Read the model definition and answer for the solid it produces. Units are mm, in the model's axes. Face numbers are marked on the shaded views. A direction names the side the tool comes from. Coordinates: 2 decimals unless noted, no trailing zeros. Loops run counter-clockwise (first coordinate to the right, second up) from the corner with the lowest first, then second, coordinate; pieces in that order, holes last. Notation, with made-up numbers: (19, -37.5) -> (60, -37.5) arc R23 cw to (60, -29.5) -> close; hole circle Ø10 at (33, 67.5). An arc over 180 degrees is marked (long way). One line per question, with ' | ' between items. Start each with the question number.
```python
from build123d import *

# Parameters (mm, degrees)
SKETCH_2_W          = 50
SKETCH_2_H          = 25
EXTRUDE_4_DEPTH     = 5
SKETCH_7_W          = 50
SKETCH_7_H          = 5
EXTRUDE_5_DEPTH     = 40.339506062
FILLET_11_R         = 2
FILLET_12_R         = 2
FILLET_15_R         = 5
FILLET_17_R         = 2
FILLET_18_R         = 2
FILLET_19_R         = 2
SKETCH_8_R          = 8.1
CUT_EXTRUDE_4_DEPTH = 25


with BuildPart() as part:
    # 草图2 → 凸台-拉伸4 (new body)
    with BuildSketch(Plane(origin=(0, 0, 0), x_dir=(1, 0, 0), z_dir=(0, 1, 0))):
        with Locations((25, 12.5)):
            Rectangle(SKETCH_2_W, SKETCH_2_H)
    extrude(amount=EXTRUDE_4_DEPTH)

    # 草图7 → 凸台-拉伸5 (add)
    with BuildSketch(Plane(origin=(0, 5, 0), x_dir=(1, 0, 0), z_dir=(0, 1, 0))):
        with Locations((25, 2.5)):
            Rectangle(SKETCH_7_W, SKETCH_7_H)
    extrude(amount=EXTRUDE_5_DEPTH)

    # 圆角11
    fillet_11_edges = [part.edges().sort_by_distance(p)[0] for p in [
        (25, 45.339506062, 0),
    ]]
    fillet(fillet_11_edges, radius=FILLET_11_R)

    # 圆角12
    fillet_12_edges = [part.edges().sort_by_distance(p)[0] for p in [
        (25, 45.339506062, -5),
    ]]
    fillet(fillet_12_edges, radius=FILLET_12_R)

    # 圆角15
    fillet_15_edges = [part.edges().sort_by_distance(p)[0] for p in [
        (25, 5, -5),
    ]]
    fillet(fillet_15_edges, radius=FILLET_15_R)

    # 圆角17
    fillet_17_edges = [part.edges().sort_by_distance(p)[0] for p in [
        (50, 45.339506062, -2.5),
        (50, 21.669753031, 0),
        (50, 44.753719625, -0.585786438),
        (50, 26.669753031, -5),
        (50, 44.753719625, -4.414213562),
        (50, 5, -17.5),
        (50, 6.464466094, -6.464466094),
        (50, 0, -12.5),
        (50, 2.5, -25),
    ]]
    fillet(fillet_17_edges, radius=FILLET_17_R)

    # 圆角18
    # the kernel refuses this fillet: 2 mm, written as the material it takes off along each edge
    with BuildSketch(Plane(origin=(48, 3, -23), x_dir=(0, 0, -1), z_dir=(0, 1, 0))) as fillet_18_piece_1_section:
        Polygon((0, 0), (FILLET_18_R, 0), (FILLET_18_R, -FILLET_18_R), (0, -FILLET_18_R), align=None)
    fillet_18_piece_1 = extrude(amount=FILLET_18_R, mode=Mode.PRIVATE)
    fillet_18_piece_1 = fillet_18_piece_1 - Plane(origin=(48, 3, -23), x_dir=(-0.7071067811865475, 0, 0.7071067811865475), z_dir=(0, 1, 0)) * Sphere(FILLET_18_R, mode=Mode.PRIVATE)
    add(fillet_18_piece_1, mode=Mode.SUBTRACT)
    with BuildSketch(Plane(origin=(48, 5, -25), x_dir=(0, 0, 1), z_dir=(-1, 0, 0))) as fillet_18_piece_2:
        with BuildLine():
            CenterArc((FILLET_18_R, -FILLET_18_R), FILLET_18_R, 90, 90)
            Line((0, -FILLET_18_R), (0, 0))
            Line((0, 0), (FILLET_18_R, 0))
        make_face()
    extrude(amount=53, mode=Mode.SUBTRACT)

    # 圆角19
    fillet_19_edges = [part.edges().sort_by_distance(p)[0] for p in [
        (0, 21.669753031, 0),
        (0, 44.753719625, -0.585786438),
        (0, 45.339506062, -2.5),
        (0, 26.669753031, -5),
        (0, 44.753719625, -4.414213562),
        (0, 6.464466094, -6.464466094),
        (0, 0, -12.5),
        (0, 5, -16.5),
        (0, 1.5, -25),
        (0, 4.414213562, -24.414213562),
    ]]
    fillet(fillet_19_edges, radius=FILLET_19_R)

    # 草图8 → 切除-拉伸4 (cut)
    with BuildSketch(Plane(origin=(0, 0, -5), x_dir=(-1, 0, 0), z_dir=(0, 0, -1))):
        with Locations(Location((-37.5, 35.339506062, 0), (0, 0, 80.987548501))):
            Circle(SKETCH_8_R)
        with Locations(Location((-12.5, 35.339506062, 0), (0, 0, 80.987548501))):
            Circle(SKETCH_8_R)
    extrude(amount=-CUT_EXTRUDE_4_DEPTH, mode=Mode.SUBTRACT)


solid = part.part
```
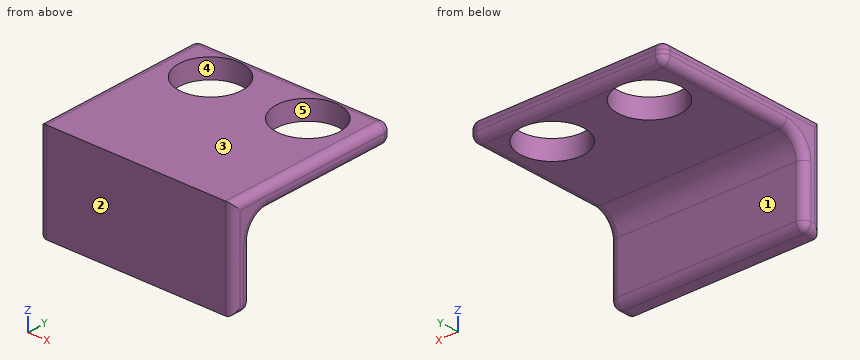
(1) Section C-C on y = 26 is taken. Write down the section's boundary in (x, z).
(2) Section A-A on x = 44.5 is taken. Write down the section's boundary in (y, z), plus the area to 3 significant figures.
(3) A tool of negligible diameter and unlimited length cuts with its end or side. For the marked faces 1 and 2, from which of +Z, -Z, +X, -X, +Y, -Y can it reach the whole face along a straight path? Write none if from no direction.
(4) Find the intervals of material crossed by probe 1 along Y at (x, z) = (12.5, -1.9); probe 2 along Z at (x, y) = (42, 28.5); probe 3 along Y at (x, z) = (29, -12.25), in increasing order. Write a range as from..to.
(5) Section D-D on y = 36 is taken. Write down the section's boundary in (x, z), plus the area to 3 significant figures.
(6) Each of these flat-tipped pins is pushed along its axis until it touches: pin 1 Ø1 at (x, z) = (41, -10.5) entering from +Y; pin 2 Ø10 at (x, y) = (15, 23) entering from -Z; pin 3 Ø6 at (x, z) = (7.5, -6.5) entering from +Y. Where does it stop, or does it pass through?
(7) Determine the mould class of the marked faces 3, 4 and 5 for opening direction X: +X half, -X half, draft (parallel to the pull), parting line (faces both ways), or undercut.
(8) Section B-B on z = -14 is taken. Write down the section's boundary in (x, y), plus the area to 3 significant figures.
Working result:
1) outline: (0, -3) arc R2 ccw to (2, -5) -> (48, -5) arc R2 ccw to (50, -3) -> (50, -2) arc R2 ccw to (48, 0) -> (2, 0) arc R2 ccw to (0, -2) -> close
2) outline: (0, -25) -> (3, -25) arc R2 ccw to (5, -23) -> (5, -10) arc R5 cw to (10, -5) -> (31.26, -5) -> (31.26, 0) -> (0, 0) -> close; (39.42, -5) -> (43.34, -5) arc R2 ccw to (45.34, -3) -> (45.34, -2) arc R2 ccw to (43.34, 0) -> (39.42, 0) -> close | area: 289 mm2
3) face 1: -Z, +X, -X, +Y | face 2: +Z, -Z, +X, -X, -Y
4) probe 1: y = 0..27.24, 43.44..45.34 | probe 2: z = -5..0 | probe 3: y = 0..5
5) outline: (0, -3) arc R2 ccw to (2, -5) -> (4.43, -5) -> (4.43, 0) -> (2, 0) arc R2 ccw to (0, -2) -> close; (20.57, -5) -> (29.43, -5) -> (29.43, 0) -> (20.57, 0) -> close; (45.57, -5) -> (48, -5) arc R2 ccw to (50, -3) -> (50, -2) arc R2 ccw to (48, 0) -> (45.57, 0) -> close | area: 85.1 mm2
6) pin 1: stops at y = 5 | pin 2: stops at z = -5 | pin 3: stops at y = 45.28
7) face 3: draft | face 4: undercut | face 5: undercut
8) outline: (0, 2) arc R2 ccw to (2, 0) -> (48, 0) arc R2 ccw to (50, 2) -> (50, 3) arc R2 ccw to (48, 5) -> (2, 5) arc R2 ccw to (0, 3) -> close | area: 247 mm2
